Could you check a few things on this drawing? It's one solid part, dimensions in mm from its lowest x, y, z. Give positions to 0.01 mm unless a question says otherwise; leave off trailing zeros. Write each loop counter-clockwise with the first axis right and the second up, starting at its lowest first coordinate (ties: lowest second). Pieces come first, ordered by that corner, then holes. Notation, with made-up numbers: (-22.75, 27.25) -> (5.25, 27.25) arc R12 ccw to (5.25, 32.25) -> close; hole circle Ø7 at (45, -10). An arc over 180 degrees is marked (long way). Answer as CSV lines item,"result". Start each with the question number.
1. If we section it at A-A on z = 50.8: Write out the boundary of the cut face in (x, y), plus the area to 3 significant figures.
2. If we section it at B-B on x = 203.2: Write out the boundary of the cut face in (y, z), plus the area to 3 significant figures.
3. I'm going to push a flat-ended pin straight in: P1, Ø10, axis at x = 203.2, z = 50.8, coming from the -Y side. Where does the tip first touch, or does it pass through?
4. I need wall thicknesses on line 1 (Z direction, x = 203.2, y = 2.5); line 2 (Z direction, x = 199.5, y = 2.5). Which ranges of each line are inside material? Lowest first, please. Write a range as [from, to].
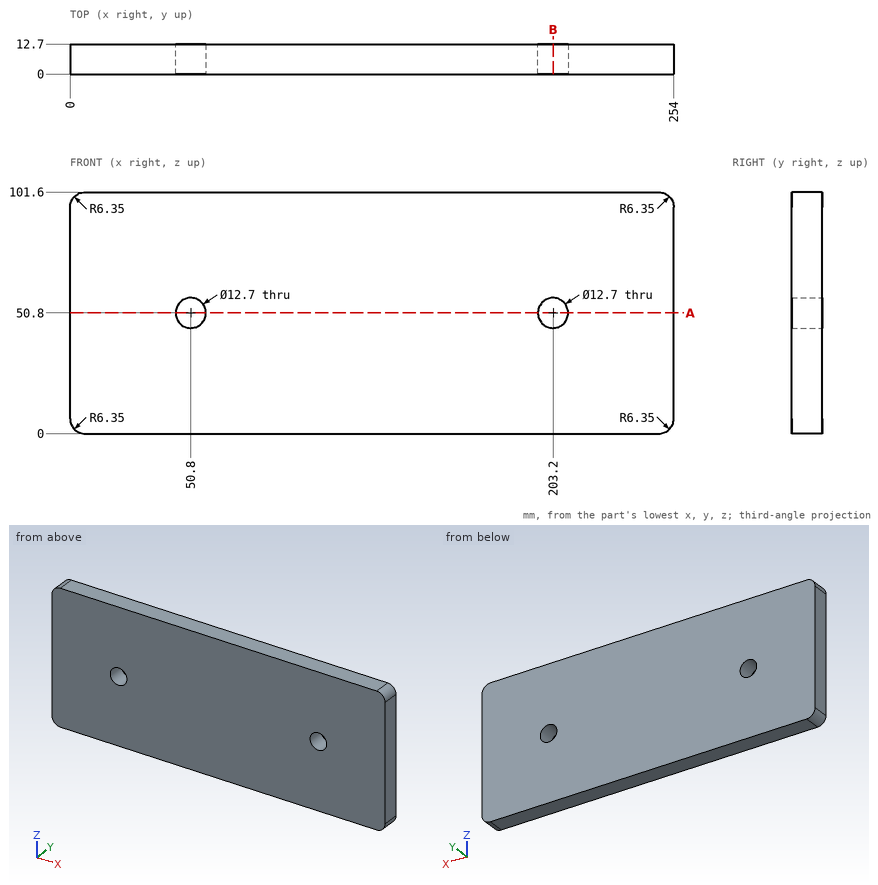
Computed values:
1,outline,"(0, 0) -> (44.45, 0) -> (44.45, 12.7) -> (0, 12.7) -> close; (57.15, 0) -> (196.85, 0) -> (196.85, 12.7) -> (57.15, 12.7) -> close; (209.55, 0) -> (254, 0) -> (254, 12.7) -> (209.55, 12.7) -> close"
1,area,"2,900 mm2"
2,outline,"(0, 0) -> (12.7, 0) -> (12.7, 44.45) -> (0, 44.45) -> close; (0, 57.15) -> (12.7, 57.15) -> (12.7, 101.6) -> (0, 101.6) -> close"
2,area,"1,130 mm2"
3,P1,"passes through"
4,line 1,"z = [0, 44.45], [57.15, 101.6]"
4,line 2,"z = [0, 45.64], [55.96, 101.6]"
